Autodesk Inventor part; units mm, degrees
ref_plane "YZ Plane" through (0, 0, 0) normal (1, 0, 0) x (0, 1, 0)
ref_plane "XZ Plane" through (0, 0, 0) normal (0, 1, 0) x (-1, 0, 0)
ref_plane "XY Plane" through (0, 0, 0) normal (0, 0, 1) x (1, 0, 0)
sketch "Skizze1" plane through (0, 0, 0) normal (0, 0, 1) x (1, 0, 0)
  line L0 (0, 0) -> (15, 0)
  line L1 (15, 0) -> (15, 4)
  line L2 (15, 4) -> (0, 4)
  line L3 (0, 4) -> (0, 0)
  dimension "d0" = 15
  dimension "d1" = 4
extrude "Extrusion1" add sketch "Skizze1" along normal blind 4
sketch "Skizze2" plane through (0, 0, 0) normal (0, -1, 0) x (1, 0, 0)
  line L0 (15, 0) -> (15, 4)
  line L1 (15, 2) -> (15, 6)
  line L2 (15, 6) -> (15, -2)
  line L3 (15, 2) -> (20, 2)
  line L4 (20, 2) -> (15, -2)
  line L5 (15, 6) -> (20, 2)
  point P0 (0, 0)
  dimension "d4" = 4
  dimension "d5" = 8
  dimension "d6" = 5
extrude "Extrusion2" add sketch "Skizze2" against normal blind 4
properties part number "ArrowUp"
The listing builds one solid part. Answer for the finished solid, in the listing's coordinates (mm). A direction names the side the tool comes from. Round coordinates to 2 decimals unless told otherwise and drop trailing zeros. Loops run counter-clockwise (first coordinate to the right, second up) from the corner with the lowest first, then second, coordinate; pieces in that order, holes last. Notation, with made-up numbers: M 22,-7.5 L 52,-7.5 A22 ccw 52,20.5 Z; hole C -8.5,-35.5 d9. An arc over 180 degrees is marked long. Return JSON: item names as keys, results as strings.
Q1. Find the intervals of material crossed by line 1 along Z through (x, y) = (12, 3.55); line 2 along X through (y, z) = (3.85, 5.75); line 3 along X through (y, z) = (1.8, 3.25), in increasing order. Write a range as from..to.
Results list:
{"line 1": "z = 0..4", "line 2": "x = 15..15.31", "line 3": "x = 0..18.44"}
Q2. Find section C-C, the plane z = 1. Determine the outline of the cut face in (x, y).
Results list:
{"outline": "M 0,0 L 18.75,0 L 18.75,4 L 0,4 Z"}
Q3. Which of the six approach directions +Z, -Z, +X, -X, +Y, -Y give full straight-line access (tool end or side, diameter ignored) to faces 1 (the face through (10, 4, 2)), 2 (the face through (7, 2, 4)), 3 (the face through (7, 2, 0))?
Results list:
{"face 1": "+Z, -Z, +X, -X, +Y", "face 2": "+Z, -X, +Y, -Y", "face 3": "-Z, -X, +Y, -Y"}
Q4. Find section A-A, the plane y = 2.7. Determine the outline of the cut face in (x, z).
Results list:
{"outline": "M 0,0 L 15,0 L 15,-2 L 20,2 L 15,6 L 15,4 L 0,4 Z"}
Q5. Each of these flat-tipped pins is pushed along its axis until it touches: pin 1 Ø0.6 at (y, z) = (2, 5.5) entering from -X; pin 2 Ø2 at (x, y) = (4, 1.5) entering from -Z; pin 3 Ø2 at (x, y) = (4.5, 3) entering from +Z. Where does it stop, or does it pass through?
Results list:
{"pin 1": "stops at x = 15", "pin 2": "stops at z = 0", "pin 3": "stops at z = 4"}
Q6. Find section B-B, the plane x = 17.25. Determine the outline of the cut face in (y, z).
Results list:
{"outline": "M 0,-0.2 L 4,-0.2 L 4,4.2 L 0,4.2 Z"}
